Print and shaded views of the part. All mm, measured from the part's lowest x, y and z. Coordinates: 2 decimals unless noted, no trailing zeros. Order: outer loops, then holes, each group sorted by start corner. A loop starts at its lowest first (then second) coordinate and runs counter-clockwise, first axis right, second up. Notation, with made-up numbers: M 80,77 L 124,77 A24 cw 124,109 Z; hole C 31.5,67 d11. An arc over 180 degrees is marked long. One line per item, written item: value.
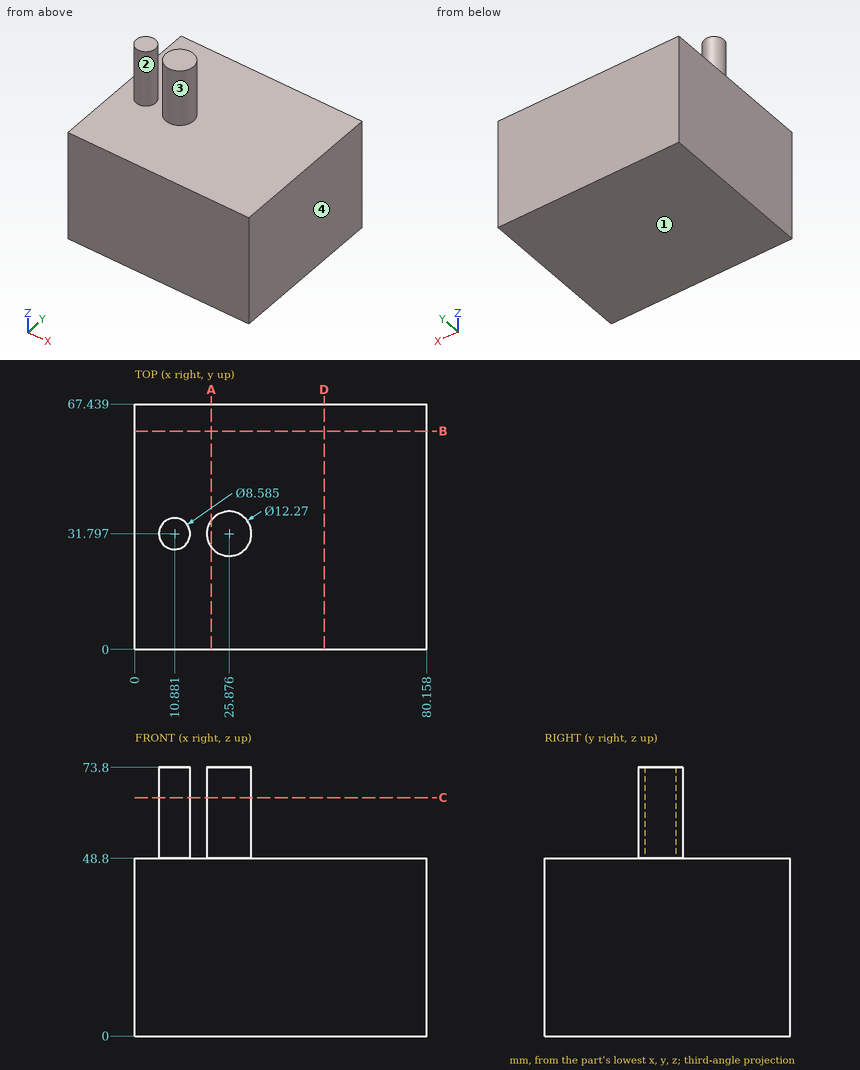
Q1. Slice it at C-C (z = 65.5). List the corners of the cut face in (x, y) (1 decimal), plus the area to 3 significant figures.
Recorded:
outline: C 10.9,31.8 d8.6; C 25.9,31.8 d12.3
area: 176 mm^2
Q2. Slice it at A-A (x = 21). List the corners of the cut face in (y, z) (1 decimal).
Recorded:
outline: M 0,0 L 67.4,0 L 67.4,48.8 L 35.5,48.8 L 35.5,73.8 L 28.1,73.8 L 28.1,48.8 L 0,48.8 Z
Q3. Drill centre lines: line 1 along Z through (x, y) = (65, 38); line 2 along Y through (x, z) = (25.5, 61.5); line 3 along X through (y, z) = (34.5, 61) (1 decimal). Where is each one in solid material? Low to high.
Recorded:
line 1: z = 0 to 48.8
line 2: y = 25.67 to 37.92
line 3: x = 7.5 to 14.2, 20.4 to 31.4
Q4. Mould opens along X. For the marked faces 1, 2, 3 and 4 say: released by +X, released by -X, zero draft, split by the parting line, or undercut.
Recorded:
face 1: zero draft
face 2: undercut
face 3: undercut
face 4: released by +X
Q5. Pin check, flat tip, straight feed: pin 1 Ø10 at (x, y) = (43, 20.5) entering from +Z. Stop position of the tip, or through.
Recorded:
pin 1: stops at z = 48.8
Q6. Slice it at B-B (y = 60). List the corners of the cut face in (x, z), plus the area to 3 significant figures.
Recorded:
outline: M 0,0 L 80.16,0 L 80.16,48.8 L 0,48.8 Z
area: 3,910 mm^2
Q7. Slice it at D-D (x = 52). List the corners of the cut face in (y, z).
Recorded:
outline: M 0,0 L 67.44,0 L 67.44,48.8 L 0,48.8 Z
